```python
from build123d import *

# Parameters (mm, degrees)
SKETCH2_R          = 2.54
CUT_EXTRUDE1_DEPTH = 63.217039467
FILLET1_R          = 2.54


with BuildPart() as part:
    # Sketch1 → Revolve1 (revolve)
    with BuildSketch(Plane(origin=(0, 0, 0), x_dir=(0, 0, -1), z_dir=(1, 0, 0))):
        Polygon((0, 0), (0, 25.4), (25.4, 25.4), (25.4, 22.225), (12.7, 9.525), (12.7, 0), align=None)
    revolve1 = revolve(axis=Axis((0, 0, 0), (0, 1, 0)))

    # Mirror1: Revolve1 across plane
    add(revolve1.mirror(Plane(origin=(0, 0, -12.7), x_dir=(0, 0, 1), z_dir=(0, -1, 0))))

    # Sketch2 → Cut-Extrude1 (cut, through all)
    with BuildSketch(Plane(origin=(0, 25.4, 0), x_dir=(1, 0, 0), z_dir=(0, 1, 0))):
        with Locations(Location((0, -16.51, 0), (0, 0, 270))):
            Circle(SKETCH2_R)
        Polygon((-7.478995387, 0), (-3.739497694, -6.477), (3.739497694, -6.477), (7.478995387, 0), (3.739497694, 6.477), (-3.739497694, 6.477), align=None)
    extrude(amount=-CUT_EXTRUDE1_DEPTH, mode=Mode.SUBTRACT)

    # Fillet1
    fillet1_edges = [part.edges().sort_by_distance(p)[0] for p in [
        (0, -22.225, 25.4),
        (0, -9.525, 12.7),
        (0, 9.525, 12.7),
        (0, 22.225, 25.4),
    ]]
    fillet(fillet1_edges, radius=FILLET1_R)


solid = part.part
```
Read the model definition and answer for the solid it produces. Units are mm, in the model's axes. A direction names the side the tool comes from. Give positions to 0.01 mm unless a question says otherwise; leave off trailing zeros. Write each loop counter-clockwise with the first axis right and the second up, starting at its lowest first coordinate (ties: lowest second). Pieces come first, ordered by that corner, then holes. Notation, with made-up numbers: M -8,-29.5 L 43,-29.5 A29 ccw 43,0.5 Z; hole C 33,49.25 d5. An arc over 180 degrees is marked long. Put each result on its own line as item: value. Start each with the question number.
1. The part is cut by section A-A, the plane y = -1. Give the vertices of the cut face in (x, z).
2. For a pull along Z with two mould halves and no side action, classify faces 4 (the flat face through (5, 25.4, 5)), 5 (the cylindrical face through (-7.629, 24.324, -24.227)), 6 (the flat face through (-5.635, 0.356, 3.193)) as released by +Z, released by -Z, zero draft, split by the parting line, or undercut.
3. The part is cut by section B-B, the plane z = 16.51. Give the number of separate pieces and of enclosed holes in the cut face, and give its area (3 significant figures).
4. Which of the six approach directions +Z, -Z, +X, -X, +Y, -Y give full straight-line access (tool end or side, diameter ignored) to faces 1 (the flat face through (5, -25.4, 5)), 2 (the flat face through (0, 0, -6.477)), 3 (the conical face through (-4.2, -10.81, -13.34))?
5. Consider line 1 along Z through (x, y) = (0, -19.25) (3 decimals); line 2 along X through (y, z) = (16, 16.51); line 3 along Y through (x, z) = (-9, 13). Determine where each line is inside the solid, lowest interval first.
6. Each of these flat-tipped pins is pushed along its axis until it touches: pin 1 Ø2 at (x, y) = (-1.5, 9) entering from +Z; pin 2 Ø2 at (x, y) = (2, -13.5) entering from +Z; pin 3 Ø3 at (y, z) = (-17.5, -18.5) entering from +X; pin 4 Ø8 at (x, z) = (0, 16.51) entering from +Y. Where does it stop, or does it pass through?
Final values:
1. outline: C 0,0 d25.4; hole M -7.48,0 L -3.74,-6.48 L 3.74,-6.48 L 7.48,0 L 3.74,6.48 L -3.74,6.48 Z
2. face 4: zero draft
2. face 5: split by the parting line
2. face 6: undercut
3. separate pieces: 4
3. enclosed holes: 0
3. area: 560 mm²
4. face 1: +Z, -Z, +X, -X, -Y
4. face 2: +Y, -Y
4. face 3: none
5. line 1: z = -22.425 to -6.477, 6.477 to 13.97, 19.05 to 22.425
5. line 2: x = -9.75 to -2.54, 2.54 to 9.75
5. line 3: y = -25.4 to -12.64, 12.64 to 25.4
6. pin 1: stops at z = 13.13
6. pin 2: stops at z = 17.45
6. pin 3: stops at x = 12.99
6. pin 4: stops at y = 25.4
